Geometry: final body of the model. Coordinates: model frame, mm. Give positions to 0.01 mm unless a question says otherwise; leave off trailing zeros. Write each loop counter-clockwise with the first axis right and the second up, starting at its lowest first coordinate (ties: lowest second). Pieces come first, ordered by that corner, then holes. Notation, with made-up numbers: (38.5, 50) -> (83.5, 50) arc R19 cw to (83.5, 80) -> close; hole circle Ø10 at (73, 37.25). An arc over 180 degrees is marked (long way). Use CSV: the item, a comma, the result in double quotes. Start each with the question number.
1) Section A-A (y = -1.2). Output: boundary loops of the cut face in (x, z) (3 decimals), plus the area to 3 significant figures.
2) Contact query for a flat-ended pin moving along its axis: P1, Ø1, axis at x = 2.5, y = -1.5, coming from the -Z side. Output: stop coordinate, or through.
3) Material intervals for line 1 (Z direction, x = -0.5, y = -0.8); line 2 (Z direction, x = -4.5, y = -2); line 3 (Z direction, x = 6, y = -0.3), sorted ascending. Write a range as [from, to].
```python
from build123d import *

# Parameters (mm, degrees)
F1_DEPTH = 3


with BuildPart() as f1:
    # F0 (on Front) → F1 (new body)
    with BuildSketch(Plane.XZ):
        with BuildLine():
            ThreePointArc((0, 100), (-5.391689, 97.766689), (-7.625, 92.375))
            Line((-7.625, 92.375), (-7.625, 0))
            Line((-7.625, 0), (-1.885, 0))
            ThreePointArc((-1.885, 0), (-1.332896, 1.332896), (0, 1.885))
            Line((0, 1.885), (0, 90.375))
            ThreePointArc((0, 90.375), (-2, 92.375), (0, 94.375))
            Line((0, 94.375), (0, 100))
        make_face()
        with BuildLine():
            ThreePointArc((7.625, 92.375), (5.391689, 97.766689), (0, 100))
            Line((0, 100), (0, 94.375))
            ThreePointArc((0, 94.375), (1.414214, 93.789214), (2, 92.375))
            ThreePointArc((2, 92.375), (1.414214, 90.960786), (0, 90.375))
            Line((0, 90.375), (0, 1.885))
            ThreePointArc((0, 1.885), (1.332896, 1.332896), (1.885, 0))
            Line((1.885, 0), (7.625, 0))
            Line((7.625, 0), (7.625, 92.375))
        make_face()
        with BuildLine():
            Line((-1.885, 0), (-7.625, 0))
            Line((-7.625, 0), (-7.625, -92.375))
            ThreePointArc((-7.625, -92.375), (-5.391689, -97.766689), (0, -100))
            Line((0, -100), (0, -94.375))
            ThreePointArc((0, -94.375), (-2, -92.375), (0, -90.375))
            Line((0, -90.375), (0, -1.885))
            ThreePointArc((0, -1.885), (-1.332896, -1.332896), (-1.885, 0))
        make_face()
        with BuildLine():
            Line((0, -94.375), (0, -100))
            ThreePointArc((0, -100), (5.391689, -97.766689), (7.625, -92.375))
            Line((7.625, -92.375), (7.625, 0))
            Line((7.625, 0), (1.885, 0))
            ThreePointArc((1.885, 0), (1.332896, -1.332896), (0, -1.885))
            Line((0, -1.885), (0, -90.375))
            ThreePointArc((0, -90.375), (1.414214, -90.960786), (2, -92.375))
            ThreePointArc((2, -92.375), (1.414214, -93.789214), (0, -94.375))
        make_face()
    extrude(amount=F1_DEPTH)


solid = f1.part
```
Answers follow:
1,outline,"(-7.625, -92.375) arc R7.625 ccw to (0, -100) arc R7.625 ccw to (7.625, -92.375) -> (7.625, 92.375) arc R7.625 ccw to (0, 100) arc R7.625 ccw to (-7.625, 92.375) -> close; hole (-1.885, 0) arc R1.885 ccw to (0, -1.885) arc R1.885 ccw to (1.885, 0) arc R1.885 ccw to (0, 1.885) arc R1.885 ccw to start; hole (0, -94.375) arc R2 ccw to (2, -92.375) arc R2 ccw to (0, -90.375) arc R2 ccw to start; hole (0, 90.375) arc R2 ccw to (2, 92.375) arc R2 ccw to (0, 94.375) arc R2 ccw to start"
1,area,"2,960 mm^2"
2,P1,"stops at z = -99.73"
3,line 1,"z = [-99.98, -94.31], [-90.44, -1.82], [1.82, 90.44], [94.31, 99.98]"
3,line 2,"z = [-98.53, 98.53]"
3,line 3,"z = [-97.08, 97.08]"
